The drawing under review shows one solid part. Ordinate dimensions are in mm from its lowest x, y, z. A direction names the side the tool comes from. Coordinates: 2 decimals unless noted, no trailing zeros. Write each loop counter-clockwise with the first axis right and the second up, starting at its lowest first coordinate (ties: lowest second). Pieces come first, ordered by that corner, then holes.
Q1. Add section D-D, the plane x = 25.5. Give the boundary of the cut face in (y, z), plus the area to 3 significant figures.
Q2. Clearance check with flat-ended pins moving along their axes: pin 1 Ø6 at (y, z) = (2.5, 6) entering from -X; pin 2 Ø3 at (x, z) = (6.5, 7.5) entering from +Y; pin 3 Ø4 at (x, y) = (49.5, 6.5) entering from +Z; pin 4 Ø1.5 at (x, z) = (25, 5) entering from +Y. State where each tip first meets the part, or that it passes through.
Q3. Add section A-A, the plane z = 6. Give the boundary of the cut face in (x, y).
Q4. To check wall thickness, follow probe 1 along X at (y, z) = (11.25, 5.25); probe 2 along Z at (x, y) = (4, 5.75); probe 3 along Y at (x, z) = (33, 9.75). State the ranges of each line that lie inside material, in increasing order.
Q5. The part is to be moulded in two halves that separate along X. For the marked faces 3, 4 and 5, say which applies: +X half, -X half, draft (parallel to the pull), parting line (faces both ways), or undercut.
Q6. Machinability: for the marked faces 1 and 2, which of the approach directions +Z, -Z, +X, -X, +Y, -Y give a long, thin tool a straight path to every point of the face, cutting with its end or side? Answer none if there is none.
Q7. Add section C-C, the plane x = 6.5. Give the boundary of the cut face in (y, z), plus the area to 3 significant figures.
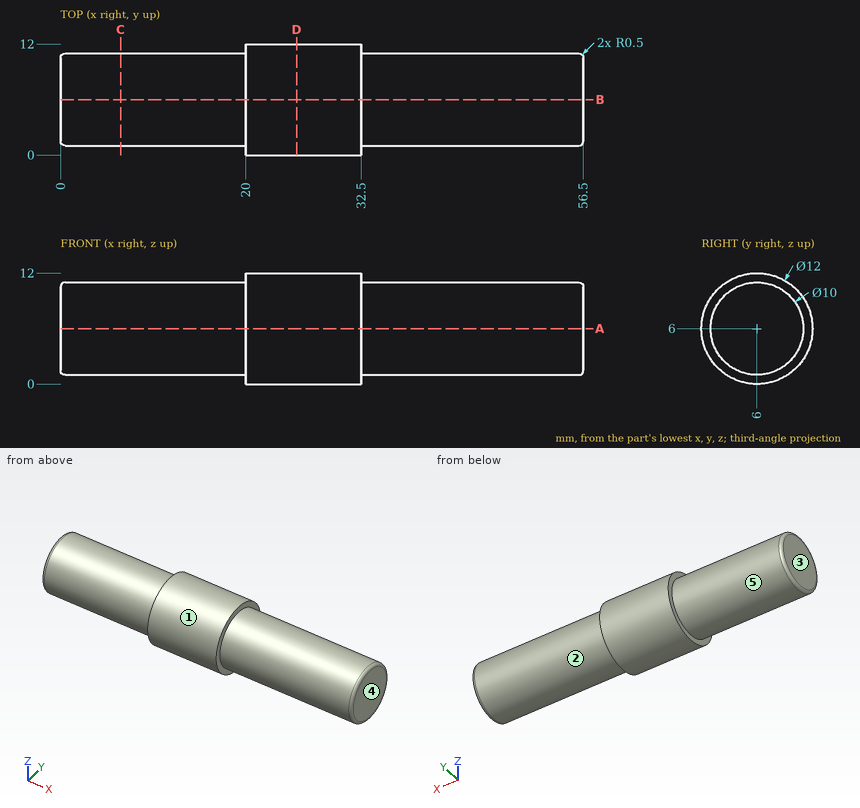
Here are the results:
1. outline: circle Ø12 at (6, 6)
1. area: 113 mm2
2. pin 1: stops at x = 0
2. pin 2: stops at y = 11
2. pin 3: stops at z = 11
2. pin 4: stops at y = 11.99
3. outline: (0, 1.5) arc R0.5 ccw to (0.5, 1) - (20, 1) - (20, 0) - (32.5, 0) - (32.5, 1) - (56, 1) arc R0.5 ccw to (56.5, 1.5) - (56.5, 10.5) arc R0.5 ccw to (56, 11) - (32.5, 11) - (32.5, 12) - (20, 12) - (20, 11) - (0.5, 11) arc R0.5 ccw to (0, 10.5) - close
4. probe 1: x = 20 to 32.5
4. probe 2: z = 1.01 to 10.99
4. probe 3: y = 2.69 to 9.31
5. face 3: -X half
5. face 4: +X half
5. face 5: draft
6. face 1: +X, -X
6. face 2: +X
7. outline: circle Ø10 at (6, 6)
7. area: 78.5 mm2
